Source: CAD feature listing. Evaluate the final solid. Frame: model axes, mm. Face numbers are marked on the shaded views. A direction names the side the tool comes from. Coordinates: 2 decimals unless noted, no trailing zeros. Loops run counter-clockwise (first coordinate to the right, second up) from the corner with the lowest first, then second, coordinate; pieces in that order, holes last.
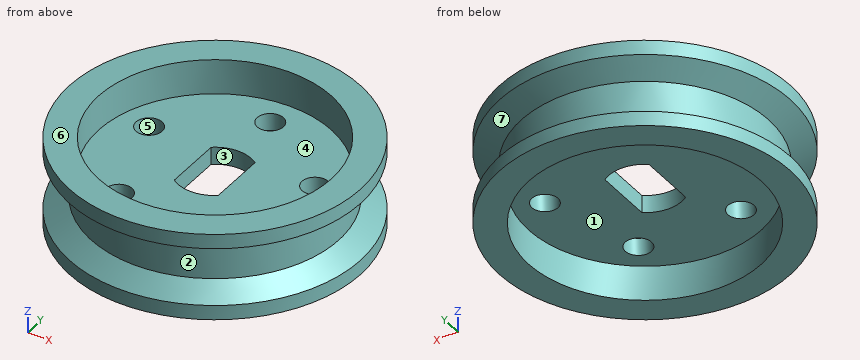
from build123d import *

# Parameters (mm, degrees)
SKETCH1_R           = 10
BOSS_EXTRUDE1_DEPTH = 3
SKETCH2_R           = 8
CUT_EXTRUDE1_DEPTH  = 2.4
SKETCH3_R           = 0.9
CUT_EXTRUDE3_DEPTH  = 4.6


with BuildPart() as part:
    # Sketch1 → Boss-Extrude1 (new body, symmetric)
    with BuildSketch(Plane.XY):
        Circle(SKETCH1_R)
        with BuildLine():
            Line((-1.521572539, 1.983637318), (-1.521572539, -2.016362682))
            ThreePointArc((-1.521572539, -2.016362682), (-0.016245384, -2.500087973), (1.478251514, -1.983871914))
            Line((1.478251514, -1.983871914), (1.478251514, 2.016128086))
            ThreePointArc((1.478251514, 2.016128086), (-0.02707564, 2.499853378), (-1.521572539, 1.983637318))
        make_face(mode=Mode.SUBTRACT)
    extrude(amount=BOSS_EXTRUDE1_DEPTH, both=True)

    # Sketch2 → Cut-Extrude1 (cut)
    with BuildSketch(Plane.XY.offset(3)):
        Circle(SKETCH2_R)
    cut_extrude1 = extrude(amount=-CUT_EXTRUDE1_DEPTH, mode=Mode.SUBTRACT)

    # Mirror1: Cut-Extrude1 across plane
    add(cut_extrude1.mirror(Plane.XY), mode=Mode.SUBTRACT)

    # Sketch5 → Cut-Revolve1 (revolve, cut)
    with BuildSketch(Plane(origin=(0, 0, 0), x_dir=(1, 0, 0), z_dir=(0, 1, 0))):
        Polygon((-10, 2), (-8.5, 1.133974596), (-8.5, -1.133974596), (-10, -2), align=None)
    revolve(axis=Axis((0, 0, 0), (0, 0, -1)), mode=Mode.SUBTRACT)

    # Sketch3 → Cut-Extrude3 (cut, through all)
    with BuildSketch(Plane.XY.offset(0.6)):
        with Locations((-3.526711514, -4.854101966)):
            Circle(SKETCH3_R)
        with Locations((0, 6)):
            Circle(SKETCH3_R)
        with Locations((5.706339098, 1.854101966)):
            Circle(SKETCH3_R)
        with Locations((3.526711514, -4.854101966)):
            Circle(SKETCH3_R)
        with Locations((-5.706339098, 1.854101966)):
            Circle(SKETCH3_R)
    extrude(amount=-CUT_EXTRUDE3_DEPTH, mode=Mode.SUBTRACT)


solid = part.part
Q1. Section A-A, the plane y = 0. Return the cut outline in (x, z).
Q2. Section C-C, the plane z = -0.2. Return the cut outline in (x, y), plus the area to 3 significant figures.
Q3. Section D-D, the plane z = -1.4. Return the cut outline in (x, y), plus the area to 3 significant figures.
Q4. Line query: line 1 along Y through (x, z) = (0, -2.3); line 2 along Z through (x, y) = (-2.5, 3); line 3 along Y through (x, z) = (-4, 0.85). Output: solid intervals per line, ascending.
Q5. Contact query for flat-ended pins moving along their axis: pin 1 Ø3 at (x, y) = (3.53, -4.85) entering from -Z; pin 2 Ø0.6 at (y, z) = (1, 0) entering from +X; pin 3 Ø2 at (x, y) = (-6.5, 1.5) entering from +Z. Output: stop coordinate, or through.
Q6. Access query for the marked faces 1, 2, 3 and 4. Directions: +Z, -Z, +X, -X, +Y, -Y. A direction counts if a zero-diameter tool reaches every point of the face in a straight line with its end or side. Return the directions, or none.
Q7. Section B-B, the plane x = 0. Return the cut outline in (y, z).
Q8. Draft query along Y for the marked faces 5, 6 and 7. Return one class per face: +Y half, -Y half, draft (parallel to the pull), parting line (faces both ways), or undercut.
Derived:
1. outline: (-10, -3) - (-8, -3) - (-8, -0.6) - (-1.52, -0.6) - (-1.52, 0.6) - (-8, 0.6) - (-8, 3) - (-10, 3) - (-10, 2) - (-8.5, 1.13) - (-8.5, -1.13) - (-10, -2) - close; (1.48, -0.6) - (8, -0.6) - (8, -3) - (10, -3) - (10, -2) - (8.5, -1.13) - (8.5, 1.13) - (10, 2) - (10, 3) - (8, 3) - (8, 0.6) - (1.48, 0.6) - close
2. outline: circle Ø17 at (0, 0); hole circle Ø1.8 at (-5.71, 1.85); hole circle Ø1.8 at (-3.53, -4.85); hole (-1.52, -2.02) arc R2.5 ccw to (1.48, -1.98) - (1.48, 2.02) arc R2.5 ccw to (-1.52, 1.98) - close; hole circle Ø1.8 at (0, 6); hole circle Ø1.8 at (3.53, -4.85); hole circle Ø1.8 at (5.71, 1.85)
2. area: 200 mm2
3. outline: circle Ø17.92 at (0, 0); hole circle Ø16 at (0, 0)
3. area: 51.2 mm2
4. line 1: y = -10 to -8, 8 to 10
4. line 2: z = -0.6 to 0.6
4. line 3: y = -7.5 to -6.93, 6.93 to 7.5
5. pin 1: stops at z = -0.6
5. pin 2: stops at x = 8.47
5. pin 3: stops at z = 0.6
6. face 1: -Z
6. face 2: none
6. face 3: +Z, -Z
6. face 4: +Z
7. outline: (-10, -3) - (-8, -3) - (-8, -0.6) - (-2.5, -0.6) - (-2.5, 0.6) - (-8, 0.6) - (-8, 3) - (-10, 3) - (-10, 2) - (-8.5, 1.13) - (-8.5, -1.13) - (-10, -2) - close; (2.5, -0.6) - (5.1, -0.6) - (5.1, 0.6) - (2.5, 0.6) - close; (6.9, -0.6) - (8, -0.6) - (8, -3) - (10, -3) - (10, -2) - (8.5, -1.13) - (8.5, 1.13) - (10, 2) - (10, 3) - (8, 3) - (8, 0.6) - (6.9, 0.6) - close
8. face 5: undercut
8. face 6: draft
8. face 7: parting line
